from build123d import *

# Parameters (mm, degrees)
SKETCH_1_R          = 1.5
SKETCH_1_R_2        = 11.5
SKETCH_1_R_3        = 7.02
SKETCH_1_W          = 4.3
SKETCH_1_H          = 8.2
SKETCH_1_H_2        = 8.3
EXTRUDE_1_DEPTH     = 4
SKETCH_2_R          = 2
CUT_EXTRUDE_1_DEPTH = 4
FILLET_1_R          = 2


with BuildPart() as part:
    # 草图1 → 凸台-拉伸1 (new body)
    with BuildSketch(Plane.XY):
        with BuildLine():
            Line((-5.457142857, -0.095714286), (-5.457142857, 41.754285714))
            Line((-5.457142857, 41.754285714), (9.542857143, 41.754285714))
            Line((9.542857143, 41.754285714), (9.542857143, 14.904285714))
            Line((9.542857143, 14.904285714), (18.542857143, 14.904285714))
            Line((18.542857143, 14.904285714), (18.542857143, 41.754285714))
            Line((18.542857143, 41.754285714), (199.542857143, 41.754285714))
            Line((199.542857143, 41.754285714), (230.542857143, 30.904285714))
            ThreePointArc((230.542857143, 30.904285714), (261.542857143, -0.095714286), (230.542857143, -31.095714286))
            Line((230.542857143, -31.095714286), (199.556073527, -38.65591431))
            Line((199.556073527, -38.65591431), (192.746868021, -40.245714286))
            Line((192.746868021, -40.245714286), (21.365844759, -40.245714286))
            Line((21.365844759, -40.245714286), (2.692857143, -38.245714286))
            Line((2.692857143, -38.245714286), (-5.457142857, -38.245714286))
            Line((-5.457142857, -38.245714286), (-5.457142857, -0.095714286))
        make_face()
        with Locations((0.542857143, 29.904285714)):
            Circle(SKETCH_1_R, mode=Mode.SUBTRACT)
        with Locations((0.542857143, -0.095714286)):
            Circle(SKETCH_1_R, mode=Mode.SUBTRACT)
        with Locations((0.542857143, -30.095714286)):
            Circle(SKETCH_1_R, mode=Mode.SUBTRACT)
        with Locations((50.542857143, -0.095714286)):
            Circle(SKETCH_1_R_2, mode=Mode.SUBTRACT)
        with Locations((50.542857143, -14.095714286)):
            Circle(SKETCH_1_R, mode=Mode.SUBTRACT)
        with Locations((36.542857143, -0.095714286)):
            Circle(SKETCH_1_R, mode=Mode.SUBTRACT)
        with Locations((50.542857143, 13.904285714)):
            Circle(SKETCH_1_R, mode=Mode.SUBTRACT)
        with Locations((64.542857143, -0.095714286)):
            Circle(SKETCH_1_R, mode=Mode.SUBTRACT)
        with Locations((230.542857143, -0.095714286)):
            Circle(SKETCH_1_R_3, mode=Mode.SUBTRACT)
        with Locations((0.542857143, 14.904285714)):
            Rectangle(SKETCH_1_W, SKETCH_1_H, mode=Mode.SUBTRACT)
        with Locations((0.542857143, -15.145714286)):
            Rectangle(SKETCH_1_W, SKETCH_1_H_2, mode=Mode.SUBTRACT)
    extrude(amount=EXTRUDE_1_DEPTH)

    # 草图2 → 切除-拉伸1 (cut)
    with BuildSketch(Plane.XY.offset(4)):
        with Locations((27.542857143, 35.754285714)):
            Circle(SKETCH_2_R)
        with Locations((112.542857143, 35.754285714)):
            Circle(SKETCH_2_R)
        with Locations((197.542857143, 35.754285714)):
            Circle(SKETCH_2_R)
        with Locations((112.542857143, -34.245714286)):
            Circle(SKETCH_2_R)
        with Locations((197.542857143, -34.245714286)):
            Circle(SKETCH_2_R)
        with Locations((27.542857143, -34.245714286)):
            Circle(SKETCH_2_R)
        Polygon((187.542857143, -24.245714286), (140.41622539, -24.245714286), (187.542857143, 14.56445304), align=None)
        Polygon((122.542857143, 25.754285714), (169.669488896, 25.754285714), (122.542857143, -13.055881612), align=None)
        with BuildLine():
            Line((71.708867631, 8.904285714), (103.542857143, 8.904285714))
            Line((103.542857143, 8.904285714), (103.542857143, 26.754285714))
            Line((103.542857143, 26.754285714), (50.083702197, 26.754285714))
            Line((50.083702197, 26.754285714), (54.496758946, 22.561881803))
            ThreePointArc((54.496758946, 22.561881803), (64.839184682, 17.921361473), (71.708867631, 8.904285714))
        make_face()
        with BuildLine():
            Line((103.542857143, -9.095714286), (103.542857143, -26.945714286))
            Line((103.542857143, -26.945714286), (50.083702197, -26.945714286))
            Line((50.083702197, -26.945714286), (54.496758946, -22.753310375))
            ThreePointArc((54.496758946, -22.753310375), (64.839184682, -18.112790044), (71.708867631, -9.095714286))
            Line((71.708867631, -9.095714286), (103.542857143, -9.095714286))
        make_face()
        with BuildLine():
            Line((125.279005787, -19.870759717), (140.7176105, -7.15661466))
            ThreePointArc((140.7176105, -7.15661466), (144.940522965, -7.565283608), (144.531854017, -11.788196074))
            Line((144.531854017, -11.788196074), (129.093249305, -24.502341131))
            ThreePointArc((129.093249305, -24.502341131), (124.870336839, -24.093672183), (125.279005787, -19.870759717))
        make_face()
    extrude(amount=-CUT_EXTRUDE_1_DEPTH, mode=Mode.SUBTRACT)

    # 圆角1
    fillet_1_edges = [part.edges().sort_by_distance(p)[0] for p in [
        (71.708867631, 8.904285714, 2),
        (50.083702197, 26.754285714, 2),
        (103.542857143, 26.754285714, 2),
        (122.542857143, -13.055881612, 2),
        (122.542857143, 25.754285714, 2),
        (169.669488896, 25.754285714, 2),
        (187.542857143, 14.56445304, 2),
        (187.542857143, -24.245714286, 2),
        (140.41622539, -24.245714286, 2),
        (103.542857143, -26.945714286, 2),
        (50.083702197, -26.945714286, 2),
        (71.708867631, -9.095714286, 2),
        (103.542857143, -9.095714286, 2),
        (9.542857143, 41.754285714, 2),
        (18.542857143, 41.754285714, 2),
    ]]
    fillet(fillet_1_edges, radius=FILLET_1_R)


solid = part.part
Work out the finished part from the listing and answer in its coordinate system (mm). A direction names the side the tool comes from. Coordinates: 2 decimals unless noted, no trailing zeros. Loops run counter-clockwise (first coordinate to the right, second up) from the corner with the lowest first, then second, coordinate; pieces in that order, holes last. Notation, with made-up numbers: M 56,80 L 77,80 A11 cw 77,96 Z; hole C 19.5,47 d8. An arc over 180 degrees is marked long. Answer in a Markdown table with one row per item. Add a question column.
1. Find section B-B, the plane x = 158. Write down the section's boundary in (y, z), then the cut area to 3 significant figures.
2. Flat-ended cylindrical pins translate along their axes: P1, Ø2.5, axis at x = 50.54, y = 13.9, coming from the -Z side; P2, Ø1.2, axis at x = 13.5, z = 1.5, coming from the +Y side. Find the tip coordinate at first contact, or state that the pin passes through.
3. Find section C-C, the plane x = 235. Write down the section's boundary in (y, z), then the cut area to 3 significant figures.
4. Find section D-D, the plane z = 1.7. State how many separate pieces and enclosed holes the cut face has, then the cut area to 3 significant figures.
5. A tool of negligible diameter and unlimited length cuts with its end or side. For faces 1 (the flat face through (136.921, -18.056, 2.028)), 2 (the flat face through (215.27, -34.82, 1.97)), from which of +Z, -Z, +X, -X, +Y, -Y can it reach the whole face along a straight path? Write none if from no direction.
6. Consider L1, parallel to X at y = 1.5, z = 3.1; L2, parallel to Y at x = 136, z = 1.9; L3, parallel to Y at x = 77, z = 3.4. Determine where each line is inside the solid, lowest interval first.
7. Find section A-A, the plane y = 4. Write down the section's boundary in (x, z).
8. The mould has two halves that part along Y. Classify faces 3 (the cylindrical face through (64.2, -18.6, 2)), 4 (the cylindrical face through (261.535, 0.586, 1.972)), 5 (the flat face through (130, -8, 4)), 6 (the flat face through (214.826, 36.405, 1.972)): pulls with the +Y half, pulls with the -Y half, needs draft (parallel to the pull), parting line crosses it, or undercut.
Reported:
| question | item | result |
|---|---|---|
| 1 | outline | M -40.25,0 L -24.25,0 L -24.25,4 L -40.25,4 Z; M -9.76,0 L 16.14,0 L 16.14,4 L -9.76,4 Z; M 25.75,0 L 41.75,0 L 41.75,4 L 25.75,4 Z |
| 1 | area | 232 mm^2 |
| 2 | P1 | passes through |
| 2 | P2 | stops at y = 14.9 |
| 3 | outline | M -30.77,0 L -5.52,0 L -5.52,4 L -30.77,4 Z; M 5.33,0 L 30.58,0 L 30.58,4 L 5.33,4 Z |
| 3 | area | 202 mm^2 |
| 4 | separate pieces | 1 |
| 4 | enclosed holes | 22 |
| 4 | area | 16,100 mm^2 |
| 5 | face 1 | +Z, -Z |
| 5 | face 2 | +Z, -Z, +X, -Y |
| 6 | L1 | x = -5.46 to 39.15, 61.93 to 122.54, 140.22 to 171.68, 187.54 to 223.71, 237.38 to 261.5 |
| 6 | L2 | y = -40.25 to -18.81, -11.04 to -1.97, 25.75 to 41.75 |
| 6 | L3 | y = -40.25 to -26.95, -9.1 to 8.9, 26.75 to 41.75 |
| 7 | outline | M -5.46,0 L 39.8,0 L 39.8,4 L -5.46,4 Z; M 61.29,0 L 122.54,0 L 122.54,4 L 61.29,4 Z; M 143.25,0 L 174.71,0 L 174.71,4 L 143.25,4 Z; M 187.54,0 L 224.84,0 L 224.84,4 L 187.54,4 Z; M 236.24,0 L 261.27,0 L 261.27,4 L 236.24,4 Z |
| 8 | face 3 | undercut |
| 8 | face 4 | parting line crosses it |
| 8 | face 5 | needs draft |
| 8 | face 6 | pulls with the +Y half |
